```python
from build123d import *

# Parameters (mm, degrees)
SKETCH_W          = 62
SKETCH_H          = 62
PAD_DEPTH         = 100
SKETCH001_W       = 30
SKETCH001_H       = 5
SKETCH001_W_2     = 5
SKETCH001_H_2     = 30
PAD001_DEPTH      = 20
FILLET_R          = 14
SKETCH002_W       = 52
SKETCH002_H       = 52
POCKET_DEPTH      = 103
SKETCH003_R       = 1.75
POCKET001_DEPTH   = 5
SKETCH004_R       = 1.75
POCKET002_DEPTH   = 5
POCKET002_FACE8_W = 52
POCKET002_FACE8_H = 100
PAD002_DEPTH      = 2
PAD002_FACE8_W    = 50
PAD002_FACE8_H    = 100
PAD003_DEPTH      = 2
PAD003_FACE25_W   = 50
PAD003_FACE25_H   = 100
PAD004_DEPTH      = 1
PAD004_FACE24_W   = 49
PAD004_FACE24_H   = 100
PAD005_DEPTH      = 1
SKETCH005_R       = 2.1
POCKET003_DEPTH   = 6
SKETCH006_R       = 2.1
POCKET004_DEPTH   = 6
SKETCH007_W       = 30
SKETCH007_H       = 20
POCKET005_DEPTH   = 5
SKETCH008_W       = 30
SKETCH008_H       = 20
POCKET006_DEPTH   = 5
SKETCH009_R       = 2.1
POCKET007_DEPTH   = 6
SKETCH010_R       = 2.1
POCKET008_DEPTH   = 6


with BuildPart() as part:
    # Sketch → Pad (new body)
    with BuildSketch(Plane.XY):
        with Locations((31, 31)):
            Rectangle(SKETCH_W, SKETCH_H)
    extrude(amount=PAD_DEPTH)

    # Sketch001 (on Face6 of Pad) → Pad001 (join)
    with BuildSketch(Plane.XY.offset(100)):
        with Locations((32, 2.5)):
            Rectangle(SKETCH001_W, SKETCH001_H)
        with Locations((59.5, 30)):
            Rectangle(SKETCH001_W_2, SKETCH001_H_2)
    extrude(amount=PAD001_DEPTH)

    # Fillet
    fillet_edges = [part.edges().sort_by_distance(p)[0] for p in [
        (62, 0, 50),
    ]]
    fillet(fillet_edges, radius=FILLET_R)

    # Sketch002 (on Face5 of Fillet) → Pocket (cut)
    with BuildSketch(Plane.XY.offset(100)):
        with Locations((26, 36)):
            Rectangle(SKETCH002_W, SKETCH002_H)
    extrude(amount=-POCKET_DEPTH, mode=Mode.SUBTRACT)

    # Sketch003 (on Face15 of Pocket) → Pocket001 (cut)
    with BuildSketch(Plane(origin=(57, 0, 0), x_dir=(0, -1, 0), z_dir=(-1, 0, 0))):
        with Locations((-37.5, 110)):
            Circle(SKETCH003_R)
        with Locations((-22.5, 110)):
            Circle(SKETCH003_R)
    extrude(amount=-POCKET001_DEPTH, mode=Mode.SUBTRACT)

    # Sketch004 (on Face12 of Pocket001) → Pocket002 (cut)
    with BuildSketch(Plane(origin=(0, 5, 0), x_dir=(-1, 0, 0), z_dir=(0, 1, 0))):
        with Locations((-39.5, 110)):
            Circle(SKETCH004_R)
        with Locations((-24.5, 110)):
            Circle(SKETCH004_R)
    extrude(amount=-POCKET002_DEPTH, mode=Mode.SUBTRACT)

    # Pocket002 Face8 → Pad002 (add)
    with BuildSketch(Plane(origin=(52, 36, 50), x_dir=(0, 1, 0), z_dir=(-1, 0, 0))):
        Rectangle(POCKET002_FACE8_W, POCKET002_FACE8_H)
    extrude(amount=PAD002_DEPTH)

    # Pad002 Face8 → Pad003 (add)
    with BuildSketch(Plane(origin=(25, 10, 50), x_dir=(1, 0, 0), z_dir=(0, 1, 0))):
        Rectangle(PAD002_FACE8_W, PAD002_FACE8_H)
    extrude(amount=PAD003_DEPTH)

    # Pad003 Face25 → Pad004 (add)
    with BuildSketch(Plane(origin=(25, 12, 50), x_dir=(1, 0, 0), z_dir=(0, 1, 0))):
        Rectangle(PAD003_FACE25_W, PAD003_FACE25_H)
    extrude(amount=PAD004_DEPTH)

    # Pad004 Face24 → Pad005 (add)
    with BuildSketch(Plane(origin=(50, 37.5, 50), x_dir=(0, 1, 0), z_dir=(-1, 0, 0))):
        Rectangle(PAD004_FACE24_W, PAD004_FACE24_H)
    extrude(amount=PAD005_DEPTH)

    # Sketch005 (on Face4 of Pad005) → Pocket003 (cut)
    with BuildSketch(Plane(origin=(0, 0, 0), x_dir=(0, -1, 0), z_dir=(-1, 0, 0))):
        with Locations((-7, 80)):
            Circle(SKETCH005_R)
        with Locations((-7, 20)):
            Circle(SKETCH005_R)
    extrude(amount=-POCKET003_DEPTH, mode=Mode.SUBTRACT)

    # Sketch006 (on Face9 of Pocket003) → Pocket004 (cut)
    with BuildSketch(Plane(origin=(0, 62, 0), x_dir=(-1, 0, 0), z_dir=(0, 1, 0))):
        with Locations((-55, 80)):
            Circle(SKETCH006_R)
        with Locations((-55, 20)):
            Circle(SKETCH006_R)
    extrude(amount=-POCKET004_DEPTH, mode=Mode.SUBTRACT)

    # Sketch007 (on Face10 of Pocket004) → Pocket005 (cut)
    with BuildSketch(Plane.YZ.offset(62)):
        with Locations((30, 10)):
            Rectangle(SKETCH007_W, SKETCH007_H)
    extrude(amount=-POCKET005_DEPTH, mode=Mode.SUBTRACT)

    # Sketch008 (on Face1 of Pocket005) → Pocket006 (cut)
    with BuildSketch(Plane.XZ):
        with Locations((32, 10)):
            Rectangle(SKETCH008_W, SKETCH008_H)
    extrude(amount=-POCKET006_DEPTH, mode=Mode.SUBTRACT)

    # Sketch009 (on Face15 of Pocket006) → Pocket007 (cut)
    with BuildSketch(Plane.YZ.offset(57)):
        with Locations((37.5, 10)):
            Circle(SKETCH009_R)
        with Locations((22.5, 10)):
            Circle(SKETCH009_R)
    extrude(amount=-POCKET007_DEPTH, mode=Mode.SUBTRACT)

    # Sketch010 (on Face17 of Pocket007) → Pocket008 (cut)
    with BuildSketch(Plane.XZ.offset(-5)):
        with Locations((39.5, 10)):
            Circle(SKETCH010_R)
        with Locations((24.5, 10)):
            Circle(SKETCH010_R)
    extrude(amount=-POCKET008_DEPTH, mode=Mode.SUBTRACT)


solid = part.part
```
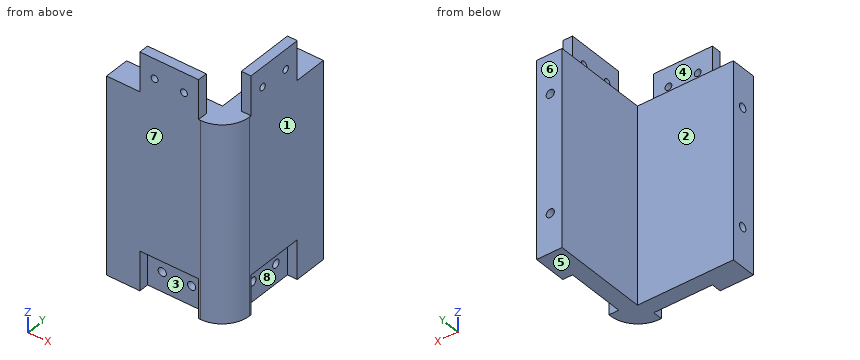
Input: part model. Units: mm. Frame: model coordinates. Face numbers are marked on the shaded views. A direction names the side the tool comes from. Give positions to 0.01 mm unless a question says otherwise; leave off trailing zeros. Order: outer loops, then holes, each group sorted by start corner. A loop starts at its lowest first (then second) coordinate and runs counter-clockwise, first axis right, second up.
1. Cut plane A-A (z = 107). Return loops of the section in (x, y), and give its area (3 significant figures).
Computed:
outline: (17, 0) - (47, 0) - (47, 5) - (17, 5) - close; (57, 15) - (62, 15) - (62, 45) - (57, 45) - close
area: 300 mm2
2. Set-up query: the marked faces 1, 2, 3 and 4. Return all of +Z, -Z, +X, -X, +Y, -Y with unobstructed straight access to the full face (end or side cutting, diameter ignored); none if empty.
Computed:
face 1: +Z, -Z, +X, +Y, -Y
face 2: +Z, -Z, -X, +Y
face 3: -Z, -Y
face 4: +Z, +X, -X, +Y
3. Pin query (flat end, axial travel): pin 1 Ø3.5 at (x, z) = (55, 20) entering from +Y; pin 2 Ø1.5 at (x, y) = (50, 53.5) entering from -Z; pin 3 Ø1.3 at (y, z) = (7, 20.5) entering from -X; pin 4 Ø12 at (x, y) = (49, 24) entering from +Z. Return the tip coordinate at first contact, or that it passes through.
Computed:
pin 1: stops at y = 56
pin 2: stops at z = 0
pin 3: stops at x = 6
pin 4: stops at z = 100
4. Draft query along Y for the marked faces 5, 6, 7 and 8. Return one class per face: released by +Y, released by -Y, zero draft, split by the parting line, or undercut.
Computed:
face 5: zero draft
face 6: released by +Y
face 7: released by -Y
face 8: undercut
5. Line query: probe 1 along X at (y, z) = (2.9, 110); probe 2 along Z at (x, y) = (55, 59); probe 3 along Y at (x, z) = (59.25, 110). Output: solid intervals per line, ascending.
Computed:
probe 1: x = 17 to 22.75, 26.25 to 37.75, 41.25 to 47
probe 2: z = 0 to 17.9, 22.1 to 77.9, 82.1 to 100
probe 3: y = 15 to 20.75, 24.25 to 35.75, 39.25 to 45
6. Cut plane D-D (z = 71). Return loops of the section in (x, y), and give its area (3 significant figures).
Computed:
outline: (0, 0) - (48, 0) arc R14 ccw to (62, 14) - (62, 62) - (49, 62) - (49, 13) - (0, 13) - close
area: 1,400 mm2
7. Cut plane C-C (x = 39.5). Return loops of the section in (y, z).
Computed:
outline: (0, 20) - (5, 20) - (5, 12.1) - (11, 12.1) - (11, 7.9) - (5, 7.9) - (5, 0) - (13, 0) - (13, 100) - (5, 100) - (5, 108.25) - (0, 108.25) - close; (0, 111.75) - (5, 111.75) - (5, 120) - (0, 120) - close
8. Cut plane B-B (y = 37.5). Return loops of the section in (x, z).
Computed:
outline: (49, 0) - (57, 0) - (57, 7.9) - (51, 7.9) - (51, 12.1) - (57, 12.1) - (57, 20) - (62, 20) - (62, 108.25) - (57, 108.25) - (57, 100) - (49, 100) - close; (57, 111.75) - (62, 111.75) - (62, 120) - (57, 120) - close
